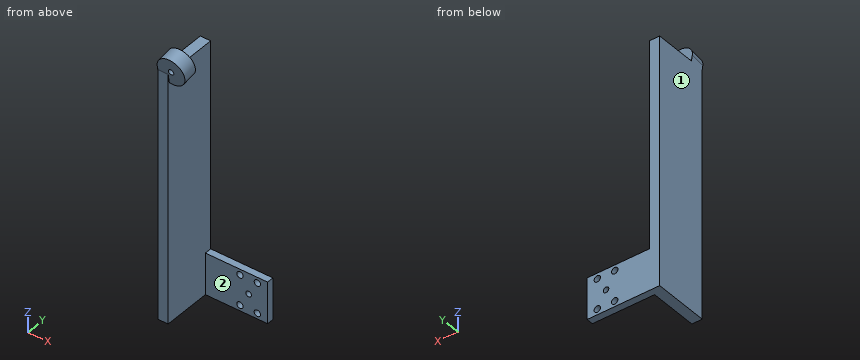
Autodesk Inventor part; units mm, degrees
ref_plane "YZ Plane" through (0, 0, 0) normal (1, 0, 0) x (0, 1, 0)
ref_plane "XZ Plane" through (0, 0, 0) normal (0, 1, 0) x (-1, 0, 0)
ref_plane "XY Plane" through (0, 0, 0) normal (0, 0, 1) x (1, 0, 0)
sketch "Sketch2" plane through (0, 0, 0) normal (1, 0, 0) x (0, 1, 0)
  line L0 (0, 0) -> (25.4, 0)
  line L1 (25.4, 0) -> (25.4, -114.3)
  line L2 (25.4, -114.3) -> (0, -114.3)
  line L3 (0, -114.3) -> (0, 0)
  dimension "d6" = 25.4
  dimension "d7" = 114.3
extrude "Extrusion2" add sketch "Sketch2" along normal blind 4.7625
sketch "Sketch3" plane through (4.7625, 0, 0) normal (1, 0, 0) x (0, 0, -1)
  line L0 (0, 0) -> (114.3, 0)
  line L1 (0, 0) -> (-14.429, -2.5442)
  line L2 (0, 0) -> (14.6516, 0) construction
  dimension "d10" = 170
ref_plane "Work Plane1" through (4.7625, -2.5442, 14.429) normal (0, 0.9848078, 0.1736482) x (0, 0.1736482, -0.9848078)
sketch "Sketch4" plane through (4.7625, -2.5442, 14.429) normal (0, 0.9848078, 0.1736482) x (0, 0.1736482, -0.9848078)
  line L0 (127.2151, 4.7625) -> (14.6516, 4.7625)
  line L1 (127.2151, 4.7625) -> (127.2151, 0)
  line L2 (14.6516, 0) -> (127.2151, 0)
  line L3 (14.6516, 4.7625) -> (14.6516, 0)
  line L4 (14.6516, 4.7625) -> (14.6516, 0)
  circle A0 centre (12.7466, -1.5875) radius 6.35
  dimension "d28" = 12.7
  dimension "d29" = 4.7625
  dimension "d30" = 1.5875
  dimension "d40" = 1.905
sketch "Sketch5" plane through (0, 25.4, 0) normal (0, 1, 0) x (1, 0, 0)
  line L0 (0, 0) -> (0, 114.3)
  line L1 (0, 0) -> (4.7625, 0)
  line L2 (4.7625, 114.3) -> (4.7625, 0)
  line L3 (0, 114.3) -> (4.7625, 114.3)
  line L4 (0, 114.3) -> (0, 0)
  line L5 (0, 114.3) -> (33.3375, 114.3)
  line L6 (33.3375, 114.3) -> (33.3375, 95.25)
  line L7 (33.3375, 95.25) -> (0, 95.25)
  line L8 (0, 95.25) -> (0, 114.3)
  dimension "d47" = 33.3375
  dimension "d48" = 4.7625
  dimension "d49" = 19.05
extrude "Extrusion4" add sketch "Sketch5" against normal blind 3.175 contours L0 L3 L2 L7 | L2 L5 L6 L7
extrude "Extrusion6" add sketch "Sketch4" along normal blind 6.35 contours A0 L2 L3 | L3 L2 A0
sketch "Sketch10" plane through (0, 0, 0) normal (-1, 0, 0) x (0, 0, 1)
  line L0 (0, 25.4) -> (-114.3, 25.4)
  line L1 (-114.3, 25.4) -> (-114.3, 0)
  line L2 (-114.3, 0) -> (0, 0)
  line L3 (0, 0) -> (0, 25.4)
  line L4 (-3.0762, 6.9904) -> (-4.1789, 0.7369)
  line L5 (0, 6.448) -> (-3.0762, 6.9904)
  line L6 (0, 0) -> (0, 6.448)
  line L7 (-4.1789, 0.7369) -> (0, 0)
  line L8 (9.2323, 4.8201) -> (-3.2748, 7.0254)
  line L9 (8.1296, -1.4335) -> (9.2323, 4.8201)
  line L10 (3.078, 5.9052) -> (1.5105, -2.9848)
  line L11 (3.078, 5.9052) -> (12.1052, 5.9052) construction
  line L12 (-114.3, 0) -> (0, 0)
  line L13 (3.078, 5.9052) -> (0, 6.448)
  line L14 (0, 0) -> (0, 25.4)
  line L15 (0, 0) -> (0, 6.448)
  line L16 (0, 0) -> (1.9753, -0.3483)
  line L17 (5.253, -0.9262) -> (-1.5008, 0.2646)
  line L18 (0, 0) -> (4.9253, -0.8685)
  point P0 (-1.1172, 0.197)
  dimension "d41" = 12.3085
  dimension "d42" = 6.1542
  dimension "d43" = 100
  dimension "d44" = 8.89
extrude "Extrusion9" add sketch "Sketch10" against normal blind 2.54
sketch "Sketch11" plane through (0, 25.4, 0) normal (0, 1, 0) x (1, 0, 0)
  line L0 (0, 0) -> (4.7625, 0)
  line L1 (4.7625, 95.25) -> (4.7625, 0)
  line L2 (4.7625, 95.25) -> (33.3375, 95.25)
  line L3 (33.3375, 95.25) -> (33.3375, 114.3)
  line L4 (0, 114.3) -> (33.3375, 114.3)
  line L5 (0, 0) -> (0, 114.3)
  circle A0 centre (24.6375, 104.775) radius 8
  line L6 (20.6375, 111.7032) -> (28.6375, 111.7032)
  line L7 (28.6375, 111.7032) -> (28.6375, 97.8468)
  line L8 (28.6375, 97.8468) -> (20.6375, 97.8468)
  line L9 (20.6375, 97.8468) -> (20.6375, 111.7032)
  point P0 (0, 0)
  dimension "d50" = 16
  dimension "d53" = 19.05
  dimension "d54" = 28.575
  dimension "d55" = 9.525
  dimension "d56" = 8
  dimension "d57" = 4
  dimension "d58" = 15.875
hole "Hole1" at (20.6375, 25.4, -111.7032) at (28.6375, 25.4, -111.7032) at (28.6375, 25.4, -97.8468) at (20.6375, 25.4, -97.8468) direction (0, -1, 0) diameter 2.921 end through all
sketch "Sketch12" plane through (0, 25.4, 0) normal (0, 1, 0) x (1, 0, 0)
  circle A0 centre (28.6375, 97.8468) radius 1.4605
  circle A1 centre (20.6375, 111.7032) radius 1.4605
  circle A2 centre (28.6375, 111.7032) radius 1.4605
  circle A3 centre (20.6375, 97.8468) radius 1.4605
  line L0 (0, 0) -> (4.7625, 0)
  line L1 (4.7625, 95.25) -> (4.7625, 0)
  line L2 (4.7625, 95.25) -> (33.3375, 95.25)
  line L3 (33.3375, 95.25) -> (33.3375, 114.3)
  line L4 (0, 114.3) -> (33.3375, 114.3)
  line L5 (0, 0) -> (0, 114.3)
  circle A4 centre (28.6375, 97.8468) radius 1.4605
  arc A5 (20.6375, 111.7032) -> (28.6375, 111.7032) centre (24.6375, 104.775) ccw
  point P0 (0, 0)
hole "Hole2" at (24.6375, 25.4, -104.775) direction (0, -1, 0) diameter 2.54 end through all
sketch "Sketch13" plane through (4.7625, 3.7093, 15.5317) normal (0, 0.9848078, 0.1736482) x (1, 0, 0)
  line L0 (-4.7625, 15.7713) -> (0, 15.7713)
  line L1 (-4.7625, 12.6458) -> (-4.7625, 15.7713)
  line L2 (-4.7625, 12.6458) -> (-4.7617, 12.6458)
  arc A0 (-4.7617, 12.6458) -> (0, 18.8949) centre (1.5875, 12.7466) ccw
  line L3 (0, 15.7713) -> (0, 18.8949)
  point P0 (-4.7625, 14.6516)
hole "Hole3" at (6.35, 5.9227, 2.9787) direction (0, -0.9848078, -0.1736482) diameter 2.54 end through all
equation "\"d30\" = 0.5 * d28 - d29"
equation "\"d42\" = 0.5 * d41"
equation "\"d55\" = 0.5 * d53"
equation "\"d57\" = 0.5 * d56"
properties part number "WheelIntakeMotorMount"
Verification items for the finished model (mm, model axes). Face numbers are marked on the shaded views. A direction names the side the tool comes from. Round coordinates to 2 decimals unless told otherwise and drop trailing zeros. Order: outer loops, then holes, each group sorted by start corner. A loop starts at its lowest first (then second) coordinate and runs counter-clockwise, first axis right, second up. Notation, with made-up numbers: (-0.5, 73) -> (50.5, 73) arc R12 ccw to (50.5, 80) -> close; hole circle Ø4 at (-28.75, 26.25). An arc over 180 degrees is marked (long way). Put each result on its own line as item: value. Start each with the question number.
(1) Section check D-D (y = 20). Enter the section's corners in (x, z), then the cut area to 3 significant figures.
(2) Depth check by flat-ended pin: pin 1 Ø1.8 at (x, z) = (20.64, -111.7) entering from +Y; pin 2 Ø2.5 at (x, y) = (3.5, 16) entering from +Z; pin 3 Ø3 at (y, z) = (12.5, -80.5) entering from +X; pin 4 Ø3 at (x, z) = (6, -80) entering from -Y. Enter the tip coordinate at first touch or a pass-through.
(3) Section check B-B (x = 11). Enter the section's corners in (y, z) (3 decimals), then the cut area to 3 significant figures.
(4) Section check A-A (z = -98). Enter the section's corners in (x, y) (1 decimal), then the cut area to 3 significant figures.
(5) Tool access check on the marked faces 1 and 2. Record the directions out of +Z, -Z, +X, -X, +Y, -Y that give a thin tool (end or side, any length) a straight path to the whole face; none if there is none.
(6) Section check C-C (z = -39.5). Enter the section's corners in (x, y), then the cut area to 3 significant figures.
(7) Material ranges on line 1 along Z through (x, y) = (21, 24.25); line 2 along X through (y, z) = (19.5, -45.5); line 3 along Y through (x, z) = (3, -109), recorded low to high.
Completed:
1. outline: (0, -114.3) -> (4.76, -114.3) -> (4.76, 0) -> (0, 0) -> close
1. area: 544 mm2
2. pin 1: passes through
2. pin 2: stops at z = 0
2. pin 3: stops at x = 4.76
2. pin 4: stops at y = 0
3. outline: (-1.082, 6.135) -> (0.42, -2.383) -> (6.674, -1.28) -> (5.172, 7.237) -> close; (22.225, -114.3) -> (25.4, -114.3) -> (25.4, -95.25) -> (22.225, -95.25) -> close
3. area: 115 mm2
4. outline: (0, 0) -> (4.8, 0) -> (4.8, 22.2) -> (19.2, 22.2) -> (19.2, 25.4) -> (0, 25.4) -> close; (22.1, 22.2) -> (27.2, 22.2) -> (27.2, 25.4) -> (22.1, 25.4) -> close; (30.1, 22.2) -> (33.3, 22.2) -> (33.3, 25.4) -> (30.1, 25.4) -> close
4. area: 193 mm2
5. face 1: +Z, -Z, -X, +Y, -Y
5. face 2: +Z, -Z, +X, -Y
6. outline: (0, 0) -> (4.76, 0) -> (4.76, 25.4) -> (0, 25.4) -> close
6. area: 121 mm2
7. line 1: z = -114.3 to -113.12, -110.29 to -99.26, -96.43 to -95.25
7. line 2: x = 0 to 4.76
7. line 3: y = 0 to 25.4
